```python
from build123d import *

# Parameters (mm, degrees)
EXTRU_MINCE1_DEPTH      = 9.5
ESQUISSE2_R             = 1.6
ENL_V_MAT_EXTRU_1_DEPTH = 30.774149862
ENL_V_START             = -2.5
ESQUISSE4_R             = 3.1
ENL_V_MAT_EXTRU_3_DEPTH = 28.274149862
SKETCH2_W               = 19
SKETCH2_H               = 8
CUT_EXTRUDE2_DEPTH      = 26.069902273
SKETCH4_W               = 19
SKETCH4_H               = 2
BOSS_EXTRUDE2_DEPTH     = 3
BOSS_EXTRUDE3_DEPTH     = 10
LPATTERN1_COUNT         = 2
LPATTERN1_PITCH         = 12
SKETCH8_R               = 1.25
CUT_EXTRUDE7_DEPTH      = 32.882597134
CUT_EXTRUDE8_DEPTH      = 32.882597134


with BuildPart() as part:
    # Esquisse1 → Extru.-Mince1 (new, symmetric)
    with BuildSketch(Plane(origin=(0, 0, 0), x_dir=(0, 0, -1), z_dir=(1, 0, 0))):
        Polygon((24.5, 0), (0, 0), (0, -14), (6, -14), (6, -6), (24.5, -6), align=None)
    extrude(amount=EXTRU_MINCE1_DEPTH, both=True)

    # Esquisse2 → Enl_v. mat.-Extru.1 (cut, through all)
    with BuildSketch(Plane(origin=(0, 0, 0), x_dir=(1, 0, 0), z_dir=(0, 1, 0))):
        with Locations(Location((0, 18, 0), (0, 0, 90))):
            Circle(ESQUISSE2_R)
    enl_v_mat_extru_1 = extrude(amount=-ENL_V_MAT_EXTRU_1_DEPTH, mode=Mode.SUBTRACT)

    # Esquisse4 → Enl_v. mat.-Extru.3 (cut, through all)
    with BuildSketch(Plane(origin=(0, 0, 0), x_dir=(1, 0, 0), z_dir=(0, 1, 0)).offset(ENL_V_START)):
        with Locations(Location((0, 18, 0), (0, 0, 270))):
            Circle(ESQUISSE4_R)
    enl_v_mat_extru_3 = extrude(amount=-ENL_V_MAT_EXTRU_3_DEPTH, mode=Mode.SUBTRACT)

    # Sketch2 → Cut-Extrude2 (cut, through all)
    with BuildSketch(Plane(origin=(0, 0, -6), x_dir=(-1, 0, 0), z_dir=(0, 0, -1))):
        with Locations((0, -10)):
            Rectangle(SKETCH2_W, SKETCH2_H)
    extrude(amount=-CUT_EXTRUDE2_DEPTH, mode=Mode.SUBTRACT)

    # Sketch4 → Boss-Extrude2 (add)
    with BuildSketch(Plane.XZ.offset(6)):
        with Locations((0, -1)):
            Rectangle(SKETCH4_W, SKETCH4_H)
        with Locations((0, -23.5)):
            Rectangle(SKETCH4_W, SKETCH4_H)
    extrude(amount=BOSS_EXTRUDE2_DEPTH)

    # Sketch5 → Boss-Extrude3 (add)
    with BuildSketch(Plane(origin=(9.5, 0, 0), x_dir=(0, 0, -1), z_dir=(1, 0, 0))):
        Polygon((0, 0), (0, -9), (2, -9), (2, -6), (22.5, -6), (22.5, -9), (24.5, -9), (24.5, 0), align=None)
    extrude(amount=BOSS_EXTRUDE3_DEPTH)

    # LPattern1: Enl_v. mat.-Extru.1, Enl_v. mat.-Extru.3 ×2
    with Locations(*[(0, 0, i * LPATTERN1_PITCH) for i in range(1, LPATTERN1_COUNT)]):
        add(enl_v_mat_extru_1, mode=Mode.SUBTRACT)
        add(enl_v_mat_extru_3, mode=Mode.SUBTRACT)

    # Sketch8 → Cut-Extrude7 (cut, through all)
    with BuildSketch(Plane.XZ.offset(6)):
        with Locations(Location((14.877046193, -17, 0), (0, 0, 270))):
            Circle(SKETCH8_R)
        with Locations(Location((14.877046193, -7.5, 0), (0, 0, 270))):
            Circle(SKETCH8_R)
    extrude(amount=-CUT_EXTRUDE7_DEPTH, mode=Mode.SUBTRACT)

    # Sketch9 → Cut-Extrude8 (cut, through all)
    with BuildSketch(Plane.XZ.offset(6)):
        with BuildLine():
            Line((14.877046193, -8.75), (8.877046193, -8.75))
            ThreePointArc((8.877046193, -8.75), (7.627046193, -7.5), (8.877046193, -6.25))
            Line((8.877046193, -6.25), (14.877046193, -6.25))
            ThreePointArc((14.877046193, -6.25), (16.127046193, -7.5), (14.877046193, -8.75))
        make_face()
        with BuildLine():
            Line((14.877046193, -18.25), (8.877046193, -18.25))
            ThreePointArc((8.877046193, -18.25), (7.627046193, -17), (8.877046193, -15.75))
            Line((8.877046193, -15.75), (14.877046193, -15.75))
            ThreePointArc((14.877046193, -15.75), (16.127046193, -17), (14.877046193, -18.25))
        make_face()
    extrude(amount=-CUT_EXTRUDE8_DEPTH, mode=Mode.SUBTRACT)


solid = part.part
```
Read the model definition and answer for the solid it produces. Units are mm, in the model's axes. A direction names the side the tool comes from. Give positions to 0.01 mm unless a question says otherwise; leave off trailing zeros. Write each loop counter-clockwise with the first axis right and the second up, starting at its lowest first coordinate (ties: lowest second). Pieces come first, ordered by that corner, then holes. Notation, with made-up numbers: (-5.75, 58.25) - (47.25, 58.25) arc R8 cw to (47.25, 70.25) - close; hole circle Ø9 at (-6, 63.25). An arc over 180 degrees is marked (long way). Write item = value, one per line. Start each with the question number.
Item 1: Find the intervals of material crossed by probe 1 along X at (y, z) = (-4.1, -6); probe 2 along Z at (x, y) = (1, -6.75); probe 3 along Z at (x, y) = (1, -2.25), in increasing order. Write a range as [from, to].
Item 2: Find section C-C (z = -4.75). Give the vertices of the cut face in (x, y).
Item 3: Find section D-D (x = -4.25). Give the vertices of the cut face in (y, z).
Item 4: A tool of negligible diameter and unlimited length cuts with its end or side. For faces 1 (the flat face through (5, -7, -22.5)), 2 (the cylindrical face through (-1.886, -4.226, -8.46)), 3 (the cylindrical face through (7.627, -3.042, -17.027)), 4 (the flat face through (5, -9, -1)), 5 (the flat face through (5, 0, -12)), from which of +Z, -Z, +X, -X, +Y, -Y can it reach the whole face along a straight path? Write none if from no direction.
Item 5: Find section A-A (y = -7). Give the vertices of the cut face in (x, z), then the cut area to 3 significant figures.
Item 6: Each of these flat-tipped pins is pushed along its axis until it touches: P1, Ø12, axis at x = 3, z = -10, coming from the -Y side; P2, Ø3, axis at x = -1.5, z = -18, coming from the -Y side. Where does it stop, or does it pass through?
Item 7: The mould has two halves that part along Z. Classify faces 6 (the flat face through (-9.5, -3, -12)), 7 (the flat face through (5, -5, -24.5)), 8 (the flat face through (5, -8, -2)): +Z half, -Z half, draft (parallel to the pull), parting line (faces both ways), or undercut.
Item 8: Find section B-B (x = 0). Give the vertices of the cut face in (y, z), then the cut area to 3 significant figures.
Response:
q1.probe_1 = [-9.5, -3.1], [3.1, 19.5]
q1.probe_2 = [-24.5, -22.5], [-2, 0]
q1.probe_3 = [-24.5, -19.25], [-16.75, -7.25], [-4.75, 0]
q2.outline = (-9.5, -6) - (-2.84, -6) - (-2.84, -2.5) - (-1, -2.5) - (-1, 0) - (-9.5, 0) - close; (1, -2.5) - (2.84, -2.5) - (2.84, -6) - (19.5, -6) - (19.5, 0) - (1, 0) - close
q3.outline = (-9, -24.5) - (0, -24.5) - (0, 0) - (-9, 0) - (-9, -2) - (-6, -2) - (-6, -22.5) - (-9, -22.5) - close
q4.face_1 = +X, -X, -Y
q4.face_2 = -Y
q4.face_3 = +Y, -Y
q4.face_4 = +Z, -Z, +X, -X, -Y
q4.face_5 = +Z, -Z, +X, -X, +Y
q5.outline = (-9.5, -24.5) - (19.5, -24.5) - (19.5, -22.5) - (-9.5, -22.5) - close; (-9.5, -2) - (19.5, -2) - (19.5, 0) - (-9.5, 0) - close
q5.area = 116 mm²
q6.P1 = -6
q6.P2 = -2.5
q7.face_6 = draft
q7.face_7 = -Z half
q7.face_8 = undercut
q8.outline = (-9, -24.5) - (0, -24.5) - (0, -19.6) - (-2.5, -19.6) - (-2.5, -21.1) - (-6, -21.1) - (-6, -22.5) - (-9, -22.5) - close; (-9, -2) - (-6, -2) - (-6, -2.9) - (-2.5, -2.9) - (-2.5, -4.4) - (0, -4.4) - (0, 0) - (-9, 0) - close; (-6, -14.9) - (-2.5, -14.9) - (-2.5, -16.4) - (0, -16.4) - (0, -7.6) - (-2.5, -7.6) - (-2.5, -9.1) - (-6, -9.1) - close
q8.area = 99.6 mm²
